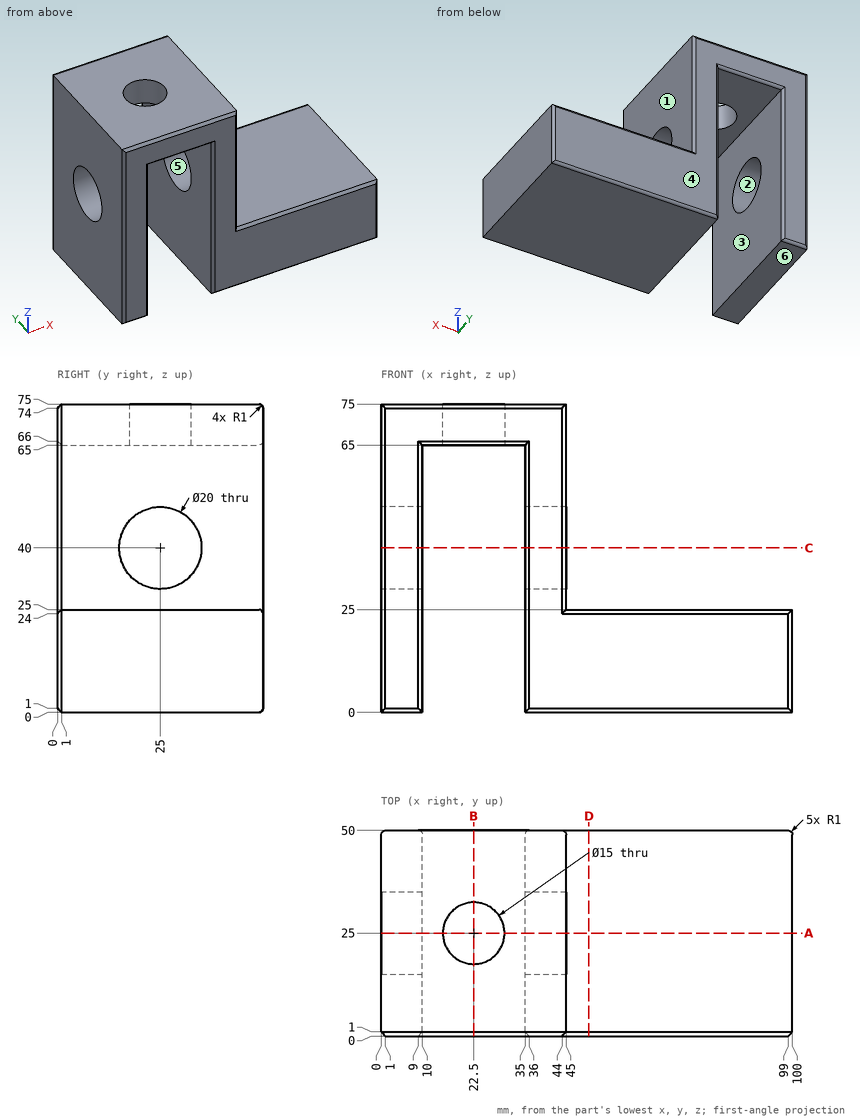
Drawing for the job (mm, zero at the part's lowest x, y, z). A direction names the side the tool comes from. Give positions to 0.01 mm unless a question says otherwise; leave off trailing zeros. Write each loop counter-clockwise with the first axis right and the second up, starting at its lowest first coordinate (ties: lowest second). Pieces come first, ordered by that corner, then holes. Notation, with made-up numbers: M 54,89 L 58,89 A28 ccw 58,121 Z; hole C -36.5,79 d11. An arc over 180 degrees is marked long. Return JSON: item names as keys, results as strings. Group by question number.
(1) Drill centre lines: L1, parallel to X at y = 35, z = 30; L2, parallel to Z at x = 42, y = 25; L3, parallel to X at y = 9.5, z = 20.5. Where is each one in solid material? Low to high. Write a range as [from, to].
(2) Band-saw the part on D-D (x = 50.5). Give the cut face in (y, z).
(3) Mould opens along Y. For the marked faces 4, 5 and 6 say: pulls with the +Y half, pulls with the -Y half, needs draft (parallel to the pull), parting line crosses it, or undercut.
(4) Band-saw the part on B-B (x = 22.5). Give the cut face in (y, z).
(5) Band-saw the part on A-A (y = 25). Give the cut face in (x, z), and give its area (4 significant figures).
(6) Flat gauge pins, fed straight in: pin 1 Ø24 at (x, y) = (73, 32) entering from +Z; pin 2 Ø12 at (x, z) = (19.5, 11.5) entering from +Y; pin 3 Ø12 at (x, z) = (15.5, 53) entering from +Y; pin 4 Ø1 at (x, y) = (31.5, 22.5) entering from -Z. Where does each tip first touch, or does it go through?
(7) 3-axis set-ups, long thin cutter, end or side, ignore diameter. For the marked faces 1, 2 and 3: which of +Z, -Z, +X, -X, +Y, -Y reach the whole face in a straight line?
(8) Band-saw the part on C-C (z = 40). Give the cut face in (x, y).
Entries:
{
 "1": {"L1": "x = [0, 10], [35, 45]", "L2": "z = [0, 30], [50, 75]", "L3": "x = [0, 10], [35, 100]"},
 "2": {"outline": "M 0,1 L 1,0 L 49,0 A1 ccw 50,1 L 50,24 A1 ccw 49,25 L 1,25 L 0,24 Z"},
 "3": {"face 4": "pulls with the +Y half", "face 5": "undercut", "face 6": "needs draft"},
 "4": {"outline": "M 0,66 L 1,65 L 17.5,65 L 17.5,75 L 1,75 L 0,74 Z; M 32.5,65 L 49,65 A1 ccw 50,66 L 50,74 A1 ccw 49,75 L 32.5,75 Z"},
 "5": {"outline": "M 0,0 L 10,0 L 10,30 L 0,30 Z; M 0,50 L 10,50 L 10,65 L 15,65 L 15,75 L 0,75 Z; M 30,65 L 35,65 L 35,50 L 45,50 L 45,75 L 30,75 Z; M 35,0 L 100,0 L 100,25 L 45,25 L 45,30 L 35,30 Z", "area": "2,575 mm^2"},
 "6": {"pin 1": "stops at z = 25", "pin 2": "passes through", "pin 3": "stops at y = 49.87", "pin 4": "stops at z = 65"},
 "7": {"face 1": "+Z, +X, +Y, -Y", "face 2": "+X, -X", "face 3": "-Z, +Y, -Y"},
 "8": {"outline": "M 0,1 L 1,0 L 9,0 L 10,1 L 10,15 L 0,15 Z; M 0,35 L 10,35 L 10,49 A1 ccw 9,50 L 1,50 A1 ccw 0,49 Z; M 35,1 L 36,0 L 44,0 L 45,1 L 45,15 L 35,15 Z; M 35,35 L 45,35 L 45,49 A1 ccw 44,50 L 36,50 A1 ccw 35,49 Z"}
}
